Here's the drawing with two shaded views (mm, measured from the low corner). I have some questions. A direction names the side the tool comes from. Coordinates: 2 decimals unless noted, no trailing zeros. Loops run counter-clockwise (first coordinate to the right, second up) from the corner with the lowest first, then second, coordinate; pieces in that order, holes last. Notation, with made-up numbers: (-9.75, 1) - (43.25, 1) arc R25 ccw to (43.25, 40) - close; hole circle Ø2 at (-6, 22.5). An arc over 180 degrees is marked (long way). Use a Markdown table: item, result.
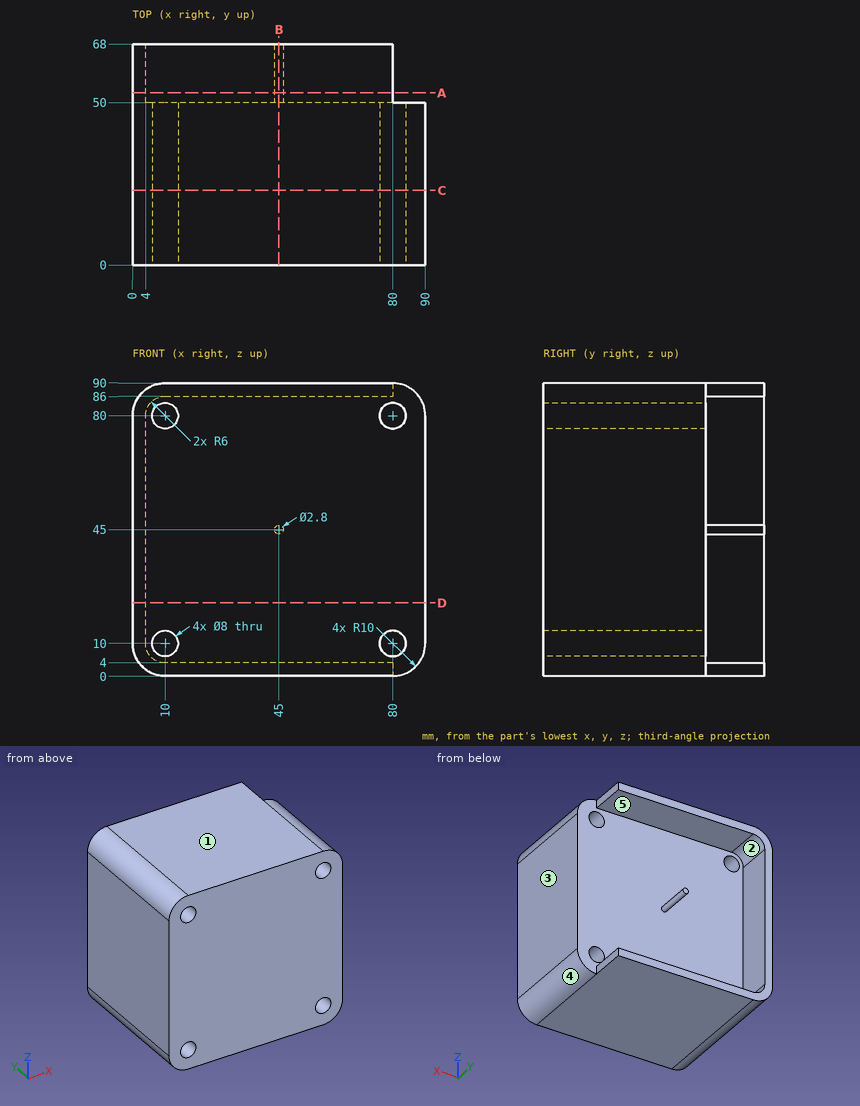
Q1. If we mould it in two halves opening along Z, with no side actions, what happens to the marked faces 3, 4 and 5? For each: pulls with the +Z half, pulls with the -Z half, needs draft (parallel to the pull), parting line crosses it, or undercut.
Check values:
| item | result |
|---|---|
| face 3 | needs draft |
| face 4 | pulls with the -Z half |
| face 5 | undercut |
Q2. Please list where these lines run through material, in increasing order: L1, parallel to Z at x = 80, y = 30; L2, parallel to Y at x = 54.5, z = 62; L3, parallel to X at y = 56, z = 43.5. Write a range as from..to.
Check values:
| item | result |
|---|---|
| L1 | 0..6, 14..76, 84..90 |
| L2 | 0..50 |
| L3 | 0..4 |
Q3. I want a section at C-C, the plane y = 23. Write out the boundary of the cut face in (x, z), then the cut area to 3 significant figures.
Check values:
| item | result |
|---|---|
| outline | (0, 10) arc R10 ccw to (10, 0) - (80, 0) arc R10 ccw to (90, 10) - (90, 80) arc R10 ccw to (80, 90) - (10, 90) arc R10 ccw to (0, 80) - close; hole circle Ø8 at (10, 10); hole circle Ø8 at (10, 80); hole circle Ø8 at (80, 10); hole circle Ø8 at (80, 80) |
| area | 7,810 mm^2 |
Q4. Which directions (+Z, -Z, +X, -X, +Y, -Y) give clear straight access to the entire face, cutting with the end or side of a thin tool? Please do the marked faces 1 and 2.
Check values:
| item | result |
|---|---|
| face 1 | +Z, +X, -X, +Y, -Y |
| face 2 | +X, +Y |
Q5. I want a section at A-A, the plane y = 53. Write out the boundary of the cut face in (x, z).
Check values:
| item | result |
|---|---|
| outline | (0, 10) arc R10 ccw to (10, 0) - (80, 0) - (80, 4) - (10, 4) arc R6 cw to (4, 10) - (4, 80) arc R6 cw to (10, 86) - (80, 86) - (80, 90) - (10, 90) arc R10 ccw to (0, 80) - close; circle Ø2.8 at (45, 45) |
Q6. Will these pins go through, and if not, where does the flat tip stop? P1, Ø3, axis at y = 60.5, z = 88.5, coming from the +X side; P2, Ø1.5, axis at y = 55, z = 57.5, coming from the +X side; P3, Ø5, axis at x = 14.5, z = 36.5, coming from the +Y side; P4, Ø6.5, axis at x = 10, z = 80, coming from the +Y side.
Check values:
| item | result |
|---|---|
| P1 | x = 80 |
| P2 | x = 4 |
| P3 | y = 50 |
| P4 | through |
Q7. I want a section at B-B, the plane x = 45. Write out the boundary of the cut face in (y, z), then the cut area to 3 significant figures.
Check values:
| item | result |
|---|---|
| outline | (0, 0) - (68, 0) - (68, 4) - (50, 4) - (50, 43.6) - (68, 43.6) - (68, 46.4) - (50, 46.4) - (50, 86) - (68, 86) - (68, 90) - (0, 90) - close |
| area | 4,690 mm^2 |
Q8. I want a section at D-D, the plane z = 22.5. Write out the boundary of the cut face in (x, y), then the cut area to 3 significant figures.
Check values:
| item | result |
|---|---|
| outline | (0, 0) - (90, 0) - (90, 50) - (4, 50) - (4, 68) - (0, 68) - close |
| area | 4,570 mm^2 |
